```python
from build123d import *

# Parameters (mm, degrees)
EXTRUDE_1_DEPTH = 15
FILLET_1_R      = 4
FILLET_2_R      = 4
FILLET_3_R      = 4


with BuildPart() as part:
    # Эскиз8 → Вытянуть-Тонкостенный1 (new body)
    with BuildSketch(Plane.XY):
        with BuildLine():
            Line((43.007359098, -6.783419957), (31.819109934, -6.783419957))
            Line((31.819109934, -6.783419957), (31.9183647, 6.609638135))
            ThreePointArc((31.9183647, 6.609638135), (0, 32.595541435), (-31.9183647, 6.609638135))
            Line((-31.9183647, 6.609638135), (-31.819109934, -6.783419957))
            Line((-31.819109934, -6.783419957), (-43.007359098, -6.783419957))
            Line((-43.007359098, -6.783419957), (-43.007359098, -7.783419957))
            Line((-43.007359098, -7.783419957), (-30.811671563, -7.783419957))
            Line((-30.811671563, -7.783419957), (-30.917598952, 6.510016405))
            ThreePointArc((-30.917598952, 6.510016405), (0, 31.595541435), (30.917598952, 6.510016405))
            Line((30.917598952, 6.510016405), (30.811671563, -7.783419957))
            Line((30.811671563, -7.783419957), (43.007359098, -7.783419957))
            Line((43.007359098, -7.783419957), (43.007359098, -6.783419957))
        make_face()
    extrude(amount=EXTRUDE_1_DEPTH)

    # Скругление1
    fillet_1_edges = [part.edges().sort_by_distance(p)[0] for p in [
        (-31.819109934, -6.783419957, 7.5),
    ]]
    fillet(fillet_1_edges, radius=FILLET_1_R)

    # Скругление2
    fillet_2_edges = [part.edges().sort_by_distance(p)[0] for p in [
        (-30.811671563, -7.783419957, 7.5),
    ]]
    fillet(fillet_2_edges, radius=FILLET_2_R)

    # Скругление3
    fillet_3_edges = [part.edges().sort_by_distance(p)[0] for p in [
        (30.811671563, -7.783419957, 7.5),
        (31.819109934, -6.783419957, 7.5),
    ]]
    fillet(fillet_3_edges, radius=FILLET_3_R)


solid = part.part
```
Work out the finished part from the listing and answer in its coordinate system (mm). A direction names the side the tool comes from. Give positions to 0.01 mm unless a question says otherwise; leave off trailing zeros. Loops run counter-clockwise (first coordinate to the right, second up) from the corner with the lowest first, then second, coordinate; pieces in that order, holes last. Notation, with made-up numbers: (89, 82) -> (120, 82) arc R23 cw to (120, 102) -> close; hole circle Ø8 at (-10.5, -29). An arc over 180 degrees is marked (long way). Put each result on its own line as item: value. Start each with the question number.
Item 1: The part is cut by section C-C (y = 28). Give the vertices of the cut face in (x, z), then the cut area to 3 significant figures.
Item 2: Find the intervals of material crossed by L1, parallel to X at y = 5.5, z = 14; L2, parallel to X at y = 28, z = 6.25; L3, parallel to Y at x = -39, z = 5, in increasing order. Write a range as [from, to].
Item 3: Each of these flat-tipped pins is pushed along its axis until it touches: P1, Ø8, axis at y = 12.5, z = 13, coming from the +X side; P2, Ø3, axis at x = 24.5, z = 6.5, coming from the +Y side; P3, Ø5.5, axis at x = 39, z = 5, coming from the +Y side. Where does it stop, or does it pass through?
Item 4: The part is cut by section D-D (x = 37). Give the vertices of the cut face in (y, z).
Item 5: The part is cut by section B-B (z = 5.25). Give the vertices of the cut face in (x, y), then the cut area to 3 significant figures.
Item 6: The mould has two halves that part along X. Classify faces 4 (the face through (32.98, -5.57, 7.6)), 5 (the face through (-32, -6.6, 7.6)), 6 (the face through (39, -7.783, 7)): released by +X, released by -X, zero draft, split by the parting line, or undercut.
Item 7: The part is cut by section A-A (y = 22). Give the vertices of the cut face in (x, z).
Item 8: Which of the six approach directions +Z, -Z, +X, -X, +Y, -Y give full straight-line access (tool end or side, diameter ignored) to faces 1 (the face through (39, -6.783, 7)), 2 (the face through (-39, -7.783, 7)), 3 (the face through (-39, -6.783, 7))?
Answers below:
1. outline: (-16.69, 0) -> (-14.64, 0) -> (-14.64, 15) -> (-16.69, 15) -> close; (14.64, 0) -> (16.69, 0) -> (16.69, 15) -> (14.64, 15) -> close
1. area: 61.5 mm2
2. L1: [-31.91, -30.91], [30.91, 31.91]
2. L2: [-16.69, -14.64], [14.64, 16.69]
2. L3: [-7.78, -6.78]
3. P1: x = 31.47
3. P2: y = 23.1
3. P3: y = -6.78
4. outline: (-7.78, 0) -> (-6.78, 0) -> (-6.78, 15) -> (-7.78, 15) -> close
5. outline: (-43.01, -7.78) -> (-34.84, -7.78) arc R4 ccw to (-30.84, -3.75) -> (-30.92, 6.51) arc R31.6 cw to (30.92, 6.51) -> (30.84, -3.75) arc R4 ccw to (34.84, -7.78) -> (43.01, -7.78) -> (43.01, -6.78) -> (35.85, -6.78) arc R4 cw to (31.85, -2.75) -> (31.92, 6.61) arc R32.6 ccw to (-31.92, 6.61) -> (-31.85, -2.75) arc R4 cw to (-35.85, -6.78) -> (-43.01, -6.78) -> close
5. area: 139 mm2
6. face 4: released by +X
6. face 5: undercut
6. face 6: zero draft
7. outline: (-24.05, 0) -> (-22.68, 0) -> (-22.68, 15) -> (-24.05, 15) -> close; (22.68, 0) -> (24.05, 0) -> (24.05, 15) -> (22.68, 15) -> close
8. face 1: +Z, -Z, +X, +Y
8. face 2: +Z, -Z, +X, -X, -Y
8. face 3: +Z, -Z, -X, +Y
